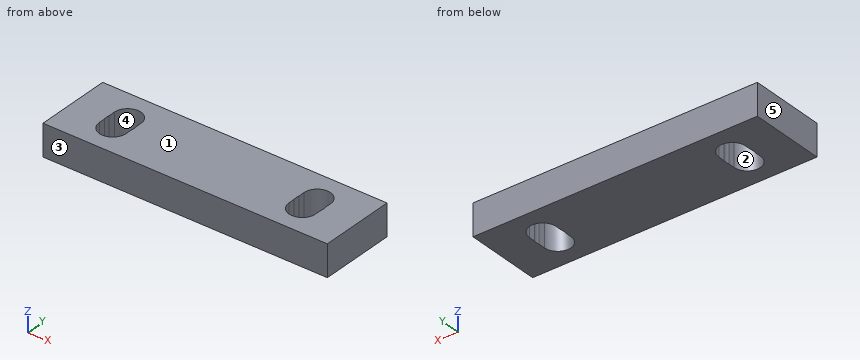
```python
from build123d import *

# Parameters (mm, degrees)
SKETCH1_W           = 45
SKETCH1_H           = 12
SKETCH1_R           = 2.15
BOSS_EXTRUDE1_DEPTH = 5
CUT_EXTRUDE1_DEPTH  = 24.817010728


with BuildPart() as part:
    # Sketch1 → Boss-Extrude1 (new body)
    with BuildSketch(Plane.XY):
        Rectangle(SKETCH1_W, SKETCH1_H)
        with Locations((-15, 0)):
            Circle(SKETCH1_R, mode=Mode.SUBTRACT)
        with Locations((15, 0)):
            Circle(SKETCH1_R, mode=Mode.SUBTRACT)
    extrude(amount=BOSS_EXTRUDE1_DEPTH)

    # Sketch2 → Cut-Extrude1 (cut, through all)
    with BuildSketch(Plane.XY.offset(5)):
        with BuildLine():
            Line((-12.9, 1.5), (-12.9, -1.5))
            ThreePointArc((-12.9, -1.5), (-15, -3.6), (-17.1, -1.5))
            Line((-17.1, -1.5), (-17.1, 1.5))
            ThreePointArc((-17.1, 1.5), (-15, 3.6), (-12.9, 1.5))
        make_face()
        with BuildLine():
            Line((12.9, -1.5), (12.9, 1.5))
            ThreePointArc((12.9, 1.5), (15, 3.6), (17.1, 1.5))
            Line((17.1, 1.5), (17.1, -1.5))
            ThreePointArc((17.1, -1.5), (15, -3.6), (12.9, -1.5))
        make_face()
    extrude(amount=-CUT_EXTRUDE1_DEPTH, mode=Mode.SUBTRACT)


solid = part.part
```
The listing builds one solid part. Answer for the finished solid, in the listing's coordinates (mm). Face numbers are marked on the shaded views. A direction names the side the tool comes from. Round coordinates to 2 decimals unless told otherwise and drop trailing zeros. Loops run counter-clockwise (first coordinate to the right, second up) from the corner with the lowest first, then second, coordinate; pieces in that order, holes last.
Q1. For a pull along Y with two mould halves and no side action, classify the marked faces 3, 4 and 5 as released by +Y, released by -Y, zero draft, split by the parting line, or undercut.
Q2. Section A-A, the plane x = 15 is taken. Determine the outline of the cut face in (y, z), then the cut area to 3 significant figures.
Q3. Find the intervals of material crossed by line 1 (X direction, y = -1.25, z = 4.35); line 2 (X direction, y = -2.5, z = 2.1); line 3 (Y direction, x = 15, z = 2.9), in increasing order.
Q4. Section C-C, the plane y = -2.5 is taken. Determine the outline of the cut face in (x, z), then the cut area to 3 significant figures.
Q5. Section D-D, the plane y = 2 is taken. Determine the outline of the cut face in (x, z), then the cut area to 3 significant figures.
Q6. Which of the six approach directions +Z, -Z, +X, -X, +Y, -Y give full straight-line access (tool end or side, diameter ignored) to the marked faces 1 and 2?
Q7. Section B-B, the plane z = 0.5 is taken. Determine the outline of the cut face in (x, y).
Completed:
1. face 3: released by -Y
1. face 4: undercut
1. face 5: zero draft
2. outline: (-6, 0) - (-3.6, 0) - (-3.6, 5) - (-6, 5) - close; (3.6, 0) - (6, 0) - (6, 5) - (3.6, 5) - close
2. area: 24.0 mm2
3. line 1: x = -22.5 to -17.1, -12.9 to 12.9, 17.1 to 22.5
3. line 2: x = -22.5 to -16.85, -13.15 to 13.15, 16.85 to 22.5
3. line 3: y = -6 to -3.6, 3.6 to 6
4. outline: (-22.5, 0) - (-16.85, 0) - (-16.85, 5) - (-22.5, 5) - close; (-13.15, 0) - (13.15, 0) - (13.15, 5) - (-13.15, 5) - close; (16.85, 0) - (22.5, 0) - (22.5, 5) - (16.85, 5) - close
4. area: 188 mm2
5. outline: (-22.5, 0) - (-17.04, 0) - (-17.04, 5) - (-22.5, 5) - close; (-12.96, 0) - (12.96, 0) - (12.96, 5) - (-12.96, 5) - close; (17.04, 0) - (22.5, 0) - (22.5, 5) - (17.04, 5) - close
5. area: 184 mm2
6. face 1: +Z, +X, -X, +Y, -Y
6. face 2: +Z, -Z
7. outline: (-22.5, -6) - (22.5, -6) - (22.5, 6) - (-22.5, 6) - close; hole (-17.1, -1.5) arc R2.1 ccw to (-12.9, -1.5) - (-12.9, -0.46) arc R2.15 ccw to (-12.9, 0.46) - (-12.9, 1.5) arc R2.1 ccw to (-17.1, 1.5) - (-17.1, 0.46) arc R2.15 ccw to (-17.1, -0.46) - close; hole (12.9, -1.5) arc R2.1 ccw to (17.1, -1.5) - (17.1, -0.46) arc R2.15 ccw to (17.1, 0.46) - (17.1, 1.5) arc R2.1 ccw to (12.9, 1.5) - (12.9, 0.46) arc R2.15 ccw to (12.9, -0.46) - close
